Here's how the part is built. I have some questions about the finished solid (model axes, mm). Face numbers are marked on the shaded views. Round coordinates to 2 decimals unless told otherwise and drop trailing zeros. Write each loop counter-clockwise with the first axis right and the second up, starting at its lowest first coordinate (ties: lowest second). Pieces come first, ordered by that corner, then holes. Notation, with made-up numbers: (41, -38) - (91, -38) arc R15 cw to (91, -25) - close; hole circle Ø1 at (-36, 86.5). An arc over 180 degrees is marked (long way). One line per question, with ' | ' between items. Start each with the question number.
(1) Imagine slicing it at A-A (y = 22.75). Write out the boundary of the cut face in (x, z).
(2) Thinking about a two-plate mould opening in Y: for the marked faces 1, 2 and 3, which applies, pulls with the +Y half, pulls with the -Y half, needs draft (parallel to the pull), parting line crosses it, or undercut?
(3) Will these pins go through, and if not, where does the flat tip stop? pin 1 (1.6 mm diameter, centred on y = 0, z = -35, fed in from +X); pin 2 (1.5 mm diameter, centred on x = 34.5, z = -50.5, fed in from +Y); pin 3 (1.8 mm diameter, centred on y = 1.5, z = -34.5, fed in from -X); pin 4 (4 mm diameter, centred on x = 6.5, y = 11.5, fed in from -Z).
(4) If I drill on L1, parallel to X at y = 1, z = -16.5; L2, parallel to Y at x = 20.5, z = -42; L3, parallel to X at y = 18.75, z = -16, over which ranges is the centre line in solid material (lowest first)?
(5) Imagine slicing it at B-B (x = 27.5). Write out the boundary of the cut face in (y, z).
(6) Imagine slicing it at C-C (z = -49). Write out the boundary of the cut face in (x, y).
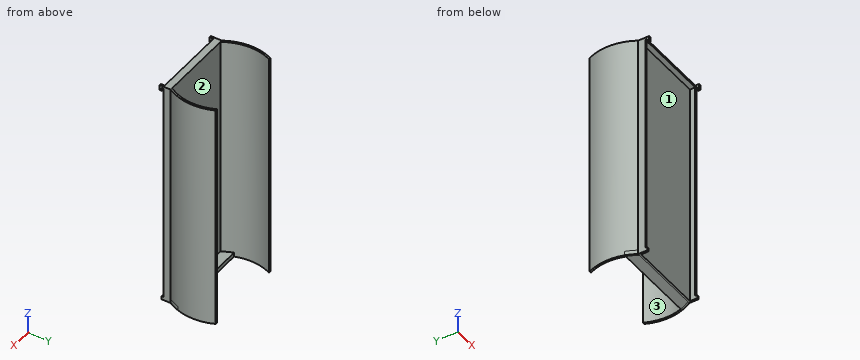
Autodesk Inventor part; units mm, degrees
ref_plane "YZ Plane" through (0, 0, 0) normal (1, 0, 0) x (0, 1, 0)
ref_plane "XZ Plane" through (0, 0, 0) normal (0, 1, 0) x (-1, 0, 0)
ref_plane "XY Plane" through (0, 0, 0) normal (0, 0, 1) x (1, 0, 0)
sketch "Sketch1" plane through (0, 0, 0) normal (0, 0, 1) x (1, 0, 0)
  line L0 (0, 0) -> (0, 2.54)
  line L1 (0, 2.54) -> (35.6964, 2.54)
  line L2 (35.6964, 2.54) -> (35.6964, 0)
  line L3 (-0.889, 0) -> (-0.889, 3.429)
  line L4 (-0.889, 3.429) -> (36.5854, 3.429)
  line L5 (36.5854, 3.429) -> (36.5854, 0)
  line L6 (-0.889, 0) -> (0, 0)
  line L7 (35.6964, 0) -> (36.5854, 0)
  line L8 (33.7232, 32.179) -> (1.9732, 32.179)
  arc A0 (36.5854, 3.429) -> (33.7232, 32.179) centre (16.0324, 15.9003) ccw
  line L9 (17.8482, 3.429) -> (17.8482, 32.179) construction
  arc A1 (1.9732, 32.179) -> (-0.889, 3.429) centre (19.664, 15.9003) ccw
  line L10 (40.0732, 15.9003) -> (-4.3768, 15.9003)
  arc A2 (35.5381, 3.429) -> (33.3287, 31.29) centre (16.0324, 15.9003) ccw
  line L11 (33.3287, 31.29) -> (2.3677, 31.29)
  arc A3 (2.3677, 31.29) -> (0.1583, 3.429) centre (19.664, 15.9003) ccw
  dimension "d0" = 35.6964
  dimension "d1" = 2.54
  dimension "d2" = 2.54
  dimension "d3" = 0.889
  dimension "d11" = 28.75
  dimension "d14" = 31.75
  dimension "d15" = 0
  dimension "d16" = 44.45
  dimension "d17" = 0.889
extrude "Extrusion1" add sketch "Sketch1" against normal blind 110 contours L6 L3 L4 L5 L7 L2 L1 L0 | A1 L10 A3 L4 | A1 L8 A0 L10 A2 L11 A3 | A2 L10 A0 L4
sketch "Sketch2" plane through (0, 0, 0) normal (0, 0, 1) x (1, 0, 0)
  line L0 (-0.889, 3.429) -> (36.5854, 3.429)
  line L1 (36.5854, 3.429) -> (36.5854, 0)
  line L2 (36.5854, 0) -> (-0.889, 0)
  line L3 (-0.889, 0) -> (-0.889, 3.429)
  line L4 (36.5854, 0) -> (36.5854, 3.429)
  line L5 (35.6964, 0) -> (36.5854, 0)
  line L6 (35.5381, 3.429) -> (0.1583, 3.429)
  line L7 (-0.889, 3.429) -> (-0.889, 0)
extrude "Extrusion2" add sketch "Sketch2" against normal blind 1
sketch "Sketch3" plane through (0, 0, -110) normal (0, 0, -1) x (-1, 0, 0)
  arc A0 (-33.7232, 32.179) -> (-36.5854, 3.429) centre (-16.0324, 15.9003) ccw
  line L0 (-37.9272, 25.829) -> (2.2308, 25.829)
  line L1 (2.2308, 25.829) -> (2.2308, 32.179)
  line L2 (2.2308, 32.179) -> (-37.9272, 32.179)
  line L3 (-37.9272, 32.179) -> (-37.9272, 25.829)
  line L4 (-1.9732, 32.179) -> (-33.7232, 32.179)
  line L5 (-17.8482, 32.179) -> (-17.8482, 3.429)
  line L6 (-35.5381, 3.429) -> (-0.1583, 3.429)
  point P0 (0, 0)
  dimension "d18" = 0
  dimension "d19" = 6.35
extrude "Extrusion3" cut sketch "Sketch3" against normal through all contours L2 L5 L0 A0 | L2 L1 L0 L5
sketch "Sketch4" plane through (0, 0, 0) normal (0, 0, 1) x (1, 0, 0)
  line L0 (35.6964, 0) -> (35.6964, 2.54)
  line L1 (35.6964, 0) -> (36.5854, 0)
  line L2 (36.5854, 0) -> (36.5854, -0.889)
  line L3 (36.5854, -0.889) -> (35.6964, -0.889)
  line L4 (35.6964, -0.889) -> (35.6964, 0)
  line L5 (36.5854, 0) -> (36.5854, 3.429)
  line L6 (0, 0) -> (-0.889, 0)
  line L7 (-0.889, 0) -> (-0.889, -0.889)
  line L8 (-0.889, -0.889) -> (0, -0.889)
  line L9 (0, -0.889) -> (0, 0)
  line L10 (-0.889, 3.429) -> (-0.889, 0)
  dimension "d23" = 0.889
  dimension "d24" = 0.889
extrude "Extrusion4" add sketch "Sketch4" against normal blind 1
sketch "Sketch5" plane through (-0.889, -0.889, 0) normal (0, -1, 0) x (1, 0, 0)
  line L0 (0.889, 0) -> (0.889, -1)
  line L1 (0, -1) -> (0, -110)
  line L2 (0.889, 0) -> (0, 0)
  line L3 (0, 0) -> (0, -2.54)
  line L4 (0, -2.54) -> (0.889, -2.54)
  line L5 (0.889, -2.54) -> (0.889, 0)
  line L6 (37.4744, 0) -> (37.4744, -110)
  line L7 (37.4744, 0) -> (36.5854, 0)
  line L8 (36.5854, 0) -> (36.5854, -2.54)
  line L9 (36.5854, -2.54) -> (37.4744, -2.54)
  line L10 (37.4744, -2.54) -> (37.4744, 0)
  line L11 (36.5854, -1) -> (36.5854, -110)
  dimension "d27" = 2.54
  dimension "d28" = 2.54
extrude "Extrusion5" add sketch "Sketch5" along normal blind 1
sketch "Sketch6" plane through (35.6964, 0, -110) normal (0, -1, 0) x (1, 0, 0)
  line L0 (0.889, 110) -> (0.889, 0)
  line L1 (0, 109) -> (0, 0)
  line L2 (0.889, 0) -> (0, 0)
  line L3 (0, 0) -> (0, 1.651)
  line L4 (0, 1.651) -> (0.889, 1.651)
  line L5 (0.889, 1.651) -> (0.889, 0)
  line L6 (-36.5854, 109) -> (-36.5854, 0)
  line L7 (-35.6964, 109) -> (-35.6964, 0)
  line L8 (-36.5854, 0) -> (-35.6964, 0)
  line L9 (-35.6964, 0) -> (-35.6964, 1.651)
  line L10 (-35.6964, 1.651) -> (-36.5854, 1.651)
  line L11 (-36.5854, 1.651) -> (-36.5854, 0)
  point P0 (-35.6964, 110)
  point P1 (-36.5854, 1.651)
  point P2 (0.889, 1.651)
  dimension "d31" = 1.651
  dimension "d32" = 1.651
extrude "Extrusion6" add sketch "Sketch6" along normal blind 1
sketch "Sketch7" plane through (0, 0, -110) normal (0, 0, -1) x (-1, 0, 0)
  arc A0 (-37.9272, 25.829) -> (-36.5854, 3.429) centre (-16.0324, 15.9003) ccw
  arc A1 (-37.9272, 25.829) -> (-36.5854, 3.429) centre (-16.0324, 15.9003) ccw
  arc A2 (0.889, 3.429) -> (2.2308, 25.829) centre (-19.664, 15.9003) ccw
  arc A3 (0.889, 3.429) -> (2.2308, 25.829) centre (-19.664, 15.9003) ccw
  line L0 (-36.5854, 3.429) -> (0.889, 3.429)
  line L1 (-35.6964, 2.54) -> (0, 2.54)
  line L2 (-38.8828, 8.429) -> (3.1864, 8.429)
  point P0 (0, 0)
  point P1 (3.1864, 8.429)
  dimension "d35" = 5
extrude "Extrusion7" add sketch "Sketch7" against normal blind 2
properties part number "PCB Battery Tray_3DPrint"
Check sheet entries:
1) outline: (-3.38, -110) - (-2.45, -110) - (-2.45, 0) - (-3.38, 0) - close; (38.15, -110) - (39.08, -110) - (39.08, 0) - (38.15, 0) - close
2) face 1: pulls with the -Y half | face 2: pulls with the +Y half | face 3: undercut
3) pin 1: x = 36.59 | pin 2: y = 3.43 | pin 3: x = -0.89 | pin 4: through
4) L1: -0.89 to 0, 35.7 to 36.59 | L2: 2.54 to 3.43 | L3: -4.21 to -3.31, 39.01 to 39.9
5) outline: (0, -1) - (2.54, -1) - (2.54, -110) - (8.43, -110) - (8.43, -108) - (3.43, -108) - (3.43, 0) - (0, 0) - close
6) outline: (-2.23, 25.83) arc R24.04 ccw to (-0.89, 3.43) - (-0.89, 0) - (0, 0) - (0, 2.54) - (35.7, 2.54) - (35.7, 0) - (36.59, 0) - (36.59, 3.43) arc R24.04 ccw to (37.93, 25.83) - (36.95, 25.83) arc R23.15 cw to (35.54, 3.43) - (0.16, 3.43) arc R23.15 cw to (-1.25, 25.83) - close
